```python
from build123d import *

# Parameters (mm, degrees)
REDONDEO1_R           = 5
REDONDEO2_R           = 2
CROQUIS2_R            = 9.525
CORTAR_EXTRUIR1_DEPTH = 60
REDONDEO3_R           = 2
CHAFL_N1_SIZE         = 5


with BuildPart() as part:
    # Croquis1 → Revolución2 (revolve)
    with BuildSketch(Plane.XY):
        Polygon((0, 175.625), (22.5, 175.625), (22.5, 115.625), (24.25, 115.625), (24.25, -31.375), (57.5, -31.375), (57.5, -166.375), (35.25, -166.375), (35.25, -46.375), (0, -46.375), align=None)
    revolve(axis=Axis((0, 96.1875, 0), (0, -1, 0)))

    # Redondeo1
    redondeo1_edges = [part.edges().sort_by_distance(p)[0] for p in [
        (-24.25, -31.375, 0),
    ]]
    fillet(redondeo1_edges, radius=REDONDEO1_R)

    # Redondeo2
    redondeo2_edges = [part.edges().sort_by_distance(p)[0] for p in [
        (-35.25, -46.375, 0),
    ]]
    fillet(redondeo2_edges, radius=REDONDEO2_R)

    # Croquis2 → Cortar-Extruir1 (cut, symmetric)
    with BuildSketch(Plane.XY):
        with Locations((0, -70.9)):
            Circle(CROQUIS2_R)
    extrude(amount=CORTAR_EXTRUIR1_DEPTH, both=True, mode=Mode.SUBTRACT)

    # Redondeo3
    redondeo3_edges = [part.edges().sort_by_distance(p)[0] for p in [
        (-57.5, -31.375, 0),
    ]]
    fillet(redondeo3_edges, radius=REDONDEO3_R)

    # Chaflán1
    chafl_n1_edges = [part.edges().sort_by_distance(p)[0] for p in [
        (-22.5, 175.625, 0),
    ]]
    chamfer(chafl_n1_edges, length=CHAFL_N1_SIZE)


solid = part.part
```
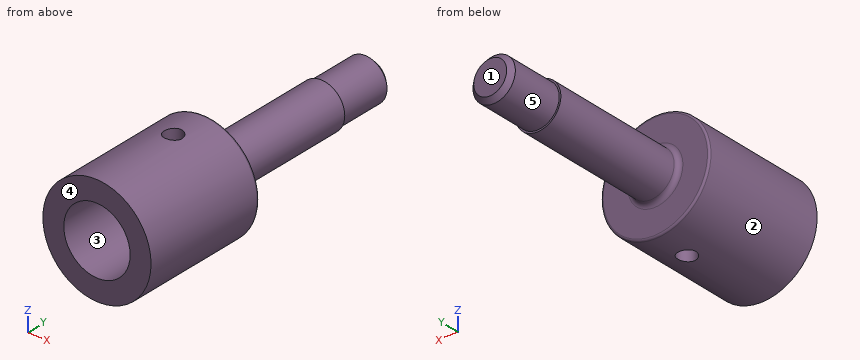
Geometry: final body of the model. Coordinates: model frame, mm. Face numbers are marked on the shaded views. A direction names the side the tool comes from. Coordinates: 2 decimals unless noted, no trailing zeros. Order: outer loops, then holes, each group sorted by start corner. A loop starts at its lowest first (then second) coordinate and runs counter-clockwise, first axis right, second up. Notation, with made-up numbers: (-35, -1.75) -> (-11, -1.75) arc R33 ccw to (-11, 32.25) -> close; hole circle Ø10 at (-19.5, 89). An arc over 180 degrees is marked (long way). Use CSV: the item, a comma, the result in double quotes.
1) Pin query (flat end, axial travel): pin 1 Ø6 at (y, z) = (125, -23.5) entering from -X; pin 2 Ø12 at (x, y) = (23.5, -94.5) entering from +Z; pin 3 Ø3 at (y, z) = (59, -5) entering from +X. Return the tip coordinate at first contact, or that it passes through.
Findings:
pin 1,"stops at x = -9.27"
pin 2,"stops at z = 54.77"
pin 3,"stops at x = 24"
2) Line query: line 1 (Y direction, x = 0, z = -50) (3 decimals); line 2 (Z direction, x = 0, y = -101); line 3 (Y direction, x = 11, z = -11) (3 decimals). Output: solid intervals per line, ascending.
Findings:
line 1,"y = -166.375 to -80.425, -61.375 to -31.375"
line 2,"z = -57.5 to -35.25, 35.25 to 57.5"
line 3,"y = -46.375 to 175.625"
3) Access query for the marked faces 4 and 5. Directions: +Z, -Z, +X, -X, +Y, -Y. A direction counts if a zero-diameter tool reaches every point of the face in a straight line with its end or side. Return the directions, or none.
Findings:
face 4,"+Z, -Z, +X, -X, -Y"
face 5,"+Y"
4) Section B-B on y = -70.9. Output: boundary loops of the cut face in (x, z) (3 decimals).
Findings:
outline,"(-9.525, -56.706) -> (-9.525, -33.939) arc R35.25 cw to (-9.525, 33.939) -> (-9.525, 56.706) arc R57.5 ccw to start; (9.525, -56.706) arc R57.5 ccw to (9.525, 56.706) -> (9.525, 33.939) arc R35.25 cw to (9.525, -33.939) -> close"
5) Mould query, pull axis Z, two halves, no side actions, for the marked faces 1, 2 and 3. Classes: +Z half, -Z half, draft (parallel to the pull), parting line (faces both ways), or undercut.
Findings:
face 1,"draft"
face 2,"parting line"
face 3,"undercut"
6) Section C-C on z = 0. Output: boundary loops of the cut face in (x, y) (3 decimals), then the cut area to 3 significant figures.
Findings:
outline,"(-57.5, -166.375) -> (-35.25, -166.375) -> (-35.25, -48.375) arc R2 cw to (-33.25, -46.375) -> (33.25, -46.375) arc R2 cw to (35.25, -48.375) -> (35.25, -166.375) -> (57.5, -166.375) -> (57.5, -33.375) arc R2 ccw to (55.5, -31.375) -> (29.25, -31.375) arc R5 cw to (24.25, -26.375) -> (24.25, 115.625) -> (22.5, 115.625) -> (22.5, 170.625) -> (17.5, 175.625) -> (-17.5, 175.625) -> (-22.5, 170.625) -> (-22.5, 115.625) -> (-24.25, 115.625) -> (-24.25, -26.375) arc R5 cw to (-29.25, -31.375) -> (-55.5, -31.375) arc R2 ccw to (-57.5, -33.375) -> close"
area,"16,900 mm^2"
7) Section D-D on y = 35.5. Output: boundary loops of the cut face in (x, z).
Findings:
outline,"circle Ø48.5 at (0, 0)"
8) Section A-A on x = 0. State how many separate pieces and enclosed holes the cut face has, then the cut area to 3 significant figures.
Findings:
separate pieces,"3"
enclosed holes,"0"
area,"16,000 mm^2"
